from build123d import *

# Parameters (mm, degrees)
ESQUISSE1_R                                        = 50
BOSS_EXTRU_1_DEPTH                                 = 61
ESQUISSE2_R                                        = 32.5
ENL_V_MAT_EXTRU_1_DEPTH                            = 19
ESQUISSE3_R                                        = 30
ENL_V_MAT_EXTRU_2_DEPTH                            = 7
ESQUISSE5_R                                        = 12.5
ENL_V_MAT_EXTRU_3_DEPTH                            = 79.89866919
CHAMBRAGE_POUR_VIS_T_TE_RONDE_BOMB_E_M_D           = 6.6
CHAMBRAGE_POUR_VIS_T_TE_RONDE_BOMB_E_M_CBORE_D     = 13
CHAMBRAGE_POUR_VIS_T_TE_RONDE_BOMB_E_M_CBORE_DEPTH = 4.6
ESQUISSE13_R                                       = 31
ENL_V_MAT_EXTRU_4_DEPTH                            = 17
ESQUISSE14_R                                       = 25.830239332
ESQUISSE14_R_2                                     = 18.153773443
ENL_V_MAT_EXTRU_5_DEPTH                            = 2
D_GAGEMENT_M61_D                                   = 6.6
D_GAGEMENT_M61_DEPTH                               = 5
D_GAGEMENT_M61_TIP                                 = 1.905255888


with BuildPart() as part:
    # Esquisse1 → Boss.-Extru.1 (new body)
    with BuildSketch(Plane.XY):
        with Locations(Location((0, 0, 0), (0, 0, 180))):
            Circle(ESQUISSE1_R)
    extrude(amount=BOSS_EXTRU_1_DEPTH)

    # Esquisse2 → Enlèv. mat.-Extru.1 (cut)
    with BuildSketch(Plane(origin=(0, 0, 0), x_dir=(-1, 0, 0), z_dir=(0, 0, -1))):
        Circle(ESQUISSE2_R)
    extrude(amount=-ENL_V_MAT_EXTRU_1_DEPTH, mode=Mode.SUBTRACT)

    # Esquisse3 → Enlèv. mat.-Extru.2 (cut)
    with BuildSketch(Plane(origin=(0, 0, 19), x_dir=(-1, 0, 0), z_dir=(0, 0, -1))):
        Circle(ESQUISSE3_R)
    extrude(amount=-ENL_V_MAT_EXTRU_2_DEPTH, mode=Mode.SUBTRACT)

    # Esquisse5 → Enlèv. mat.-Extru.3 (cut, through all)
    with BuildSketch(Plane(origin=(0, 0, 26), x_dir=(-1, 0, 0), z_dir=(0, 0, -1))):
        Circle(ESQUISSE5_R)
    extrude(amount=-ENL_V_MAT_EXTRU_3_DEPTH, mode=Mode.SUBTRACT)

    # Chambrage pour vis à tête ronde bombée M61 (through all)
    with Locations(Plane(origin=(0, 0, 0), x_dir=(-1, 0, 0), z_dir=(0, 0, -1))):
        with Locations((41.25, 0), (0, 41.25), (-41.25, 0), (0, -41.25)):
            CounterBoreHole(CHAMBRAGE_POUR_VIS_T_TE_RONDE_BOMB_E_M_D / 2, CHAMBRAGE_POUR_VIS_T_TE_RONDE_BOMB_E_M_CBORE_D / 2, CHAMBRAGE_POUR_VIS_T_TE_RONDE_BOMB_E_M_CBORE_DEPTH)

    # Esquisse13 → Enlèv. mat.-Extru.4 (cut)
    with BuildSketch(Plane.XY.offset(61)):
        Circle(ESQUISSE13_R)
    extrude(amount=-ENL_V_MAT_EXTRU_4_DEPTH, mode=Mode.SUBTRACT)

    # Esquisse14 → Enlèv. mat.-Extru.5 (cut)
    with BuildSketch(Plane.XY.offset(44)):
        Circle(ESQUISSE14_R)
        Circle(ESQUISSE14_R_2, mode=Mode.SUBTRACT)
    extrude(amount=-ENL_V_MAT_EXTRU_5_DEPTH, mode=Mode.SUBTRACT)

    # Dégagement M61
    with Locations(Plane.XY.offset(61)):
        with Locations((-23.608593004, 25.838621023), (-25.838621023, -23.608593004), (23.608593004, -25.838621023), (25.838621023, 23.608593004)):
            Hole(D_GAGEMENT_M61_D / 2, depth=D_GAGEMENT_M61_DEPTH)
            with Locations((0, 0, -(D_GAGEMENT_M61_DEPTH + D_GAGEMENT_M61_TIP / 2))):  # 120° drill point
                Cone(0, D_GAGEMENT_M61_D / 2, D_GAGEMENT_M61_TIP, mode=Mode.SUBTRACT)


solid = part.part
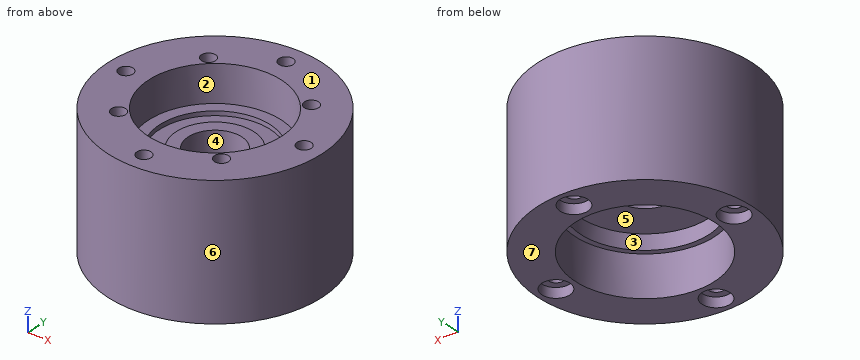
Could you check a few things on this model? Use its own coordinates, in mm. Face numbers are marked on the shaded views. A direction names the side the tool comes from. Coordinates: 2 decimals unless noted, no trailing zeros. Write each loop counter-clockwise with the first axis right and the second up, starting at its lowest first coordinate (ties: lowest second). Pieces come first, ordered by that corner, then holes. Notation, with made-up numbers: (71, 20) - (128, 20) arc R12 ccw to (128, 42) - close; hole circle Ø2 at (80.25, 25). An arc over 180 degrees is marked (long way). Put each result on its own line as item: value. Start each with the question number.
Q1. Thinking about a two-plate mould opening in X: for the marked faces 4, 5, 6 and 7, which applies, pulls with the +X half, pulls with the -X half, needs draft (parallel to the pull), parting line crosses it, or undercut?
Q2. Please list where these lines run through material, in increasing order: L1, parallel to Y at x = 0, z = 15; L2, parallel to Y at x = -3, z = 30; L3, parallel to Z at x = 12.5, y = -12.
Q3. I want a section at B-B on x = -41.25. Write out the boundary of the cut face in (y, z), plus the area to 3 significant figures.
Q4. I want a section at C-C on y = 0. Count the separate pieces of the cut face and the enclosed holes in it, plus the area to 3 significant figures.
Q5. Which directions (+Z, -Z, +X, -X, +Y, -Y) give clear straight access to the entire face, cutting with the end or side of a thin tool? Please do the marked faces 1, 2 and 3.
Q6. I want a section at A-A on z = 23. Write out the boundary of the cut face in (x, y).
Q7. I'm going to push flat-ended pins straight in: P1, Ø5, axis at x = 4.5, z = 8.5, coming from the -Y side; P2, Ø1.5, axis at y = 32.5, z = 38.5, coming from the +X side; P3, Ø5.5, axis at x = -25.84, y = -23.61, coming from the +Z side. Where does each tip first touch, or does it pass through?
Checks:
1. face 4: undercut
1. face 5: undercut
1. face 6: parting line crosses it
1. face 7: needs draft
2. L1: -50 to -44.55, -37.95 to -32.5, 32.5 to 37.95, 44.55 to 50
2. L2: -49.91 to -42.62, -39.88 to -12.13, 12.13 to 39.88, 42.62 to 49.91
2. L3: 26 to 44
3. outline: (-28.26, 0) - (-6.5, 0) - (-6.5, 4.6) - (-3.3, 4.6) - (-3.3, 61) - (-28.26, 61) - close; (3.3, 4.6) - (6.5, 4.6) - (6.5, 0) - (28.26, 0) - (28.26, 61) - (3.3, 61) - close
3. area: 3,020 mm²
4. separate pieces: 4
4. enclosed holes: 0
4. area: 2,050 mm²
5. face 1: +Z, +X, -X, +Y, -Y
5. face 2: +Z
5. face 3: -Z
6. outline: circle Ø100 at (0, 0); hole circle Ø6.6 at (-41.25, 0); hole circle Ø60 at (0, 0); hole circle Ø6.6 at (0, -41.25); hole circle Ø6.6 at (0, 41.25); hole circle Ø6.6 at (41.25, 0)
7. P1: y = -49.96
7. P2: x = 38.63
7. P3: z = 55.68
